Geometry check sheet. Reference: the model listing, model coordinates, mm. Face numbers are marked on the shaded views. A direction names the side the tool comes from. Give positions to 0.01 mm unless a question says otherwise; leave off trailing zeros. Loops run counter-clockwise (first coordinate to the right, second up) from the corner with the lowest first, then second, coordinate; pieces in that order, holes last. Notation, with made-up numbers: (15.5, 55.25) -> (58.5, 55.25) arc R16 ccw to (58.5, 69.25) -> close; hole circle Ø7 at (2.5, 76). An arc over 180 degrees is marked (long way). Answer as a JSON object with one key per item and string values.
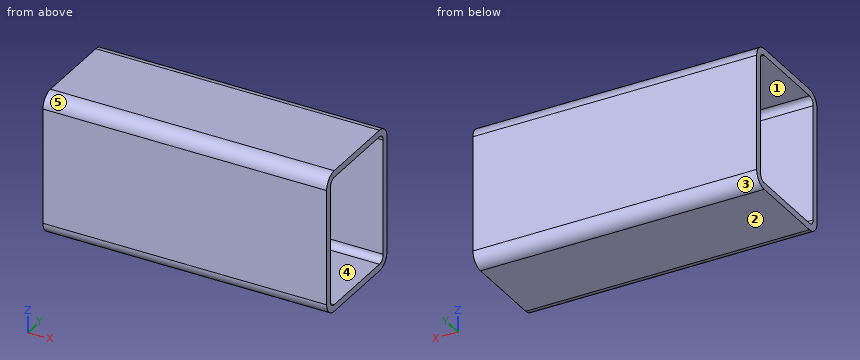
from build123d import *

# Parameters (mm, degrees)
F2_DEPTH = 101.6


# Not quite as in the source:
# - a variable given as a bare number and used for a length is read in inches; the dataset says mm whatever the document's units were


with BuildPart() as f2:
    # F1 (on Right) → F2 (new body, symmetric)
    with BuildSketch(Plane.YZ):
        with BuildLine():
            Line((28.575, 50.8), (-28.575, 50.8))
            ThreePointArc((-28.575, 50.8), (-35.3101920908, 48.0101920908), (-38.1, 41.275))
            Line((-38.1, 41.275), (-38.1, -41.275))
            ThreePointArc((-38.1, -41.275), (-35.3101920908, -48.0101920908), (-28.575, -50.8))
            Line((-28.575, -50.8), (28.575, -50.8))
            ThreePointArc((28.575, -50.8), (35.3101920908, -48.0101920908), (38.1, -41.275))
            Line((38.1, -41.275), (38.1, 41.275))
            ThreePointArc((38.1, 41.275), (35.3101920908, 48.0101920908), (28.575, 50.8))
        make_face()
        with BuildLine():
            ThreePointArc((-33.3375, 41.275), (-31.9425960454, 44.6425960454), (-28.575, 46.0375))
            Line((-28.575, 46.0375), (28.575, 46.0375))
            ThreePointArc((28.575, 46.0375), (31.9425960454, 44.6425960454), (33.3375, 41.275))
            Line((33.3375, 41.275), (33.3375, -41.275))
            ThreePointArc((33.3375, -41.275), (31.9425960454, -44.6425960454), (28.575, -46.0375))
            Line((28.575, -46.0375), (-28.575, -46.0375))
            ThreePointArc((-28.575, -46.0375), (-31.9425960454, -44.6425960454), (-33.3375, -41.275))
            Line((-33.3375, -41.275), (-33.3375, 41.275))
        make_face(mode=Mode.SUBTRACT)
    extrude(amount=F2_DEPTH, both=True)


solid = f2.part
1) Material ranges on line 1 along Y through (x, z) = (15.5, 22); line 2 along Z through (x, y) = (-57.5, -1.5); line 3 along Z through (x, y) = (6, -32), recorded low to high. Write a range as from..to.
Geometry check:
{"line 1": "y = -38.1..-33.34, 33.34..38.1", "line 2": "z = -50.8..-46.04, 46.04..50.8", "line 3": "z = -50.16..-44.58, 44.58..50.16"}
2) Depth check by flat-ended pin: P1, Ø4, axis at y = 29.5, z = -12, coming from the +X side. Enter the tip coordinate at first touch or a pass-through.
Geometry check:
{"P1": "passes through"}
3) Draft check along Y on the marked faces 1, 2 and 3. Enter one of: pulls with the +Y half, pulls with the -Y half, needs draft (parallel to the pull), parting line crosses it, or undercut.
Geometry check:
{"face 1": "undercut", "face 2": "needs draft", "face 3": "pulls with the +Y half"}
4) Section check B-B on y = -6. Record the cut outline in (x, z).
Geometry check:
{"outline": "(-101.6, -50.8) -> (101.6, -50.8) -> (101.6, -46.04) -> (-101.6, -46.04) -> close; (-101.6, 46.04) -> (101.6, 46.04) -> (101.6, 50.8) -> (-101.6, 50.8) -> close"}
5) Section check A-A on z = 16. Record the cut outline in (x, y), plus the area to 3 significant figures.
Geometry check:
{"outline": "(-101.6, -38.1) -> (101.6, -38.1) -> (101.6, -33.34) -> (-101.6, -33.34) -> close; (-101.6, 33.34) -> (101.6, 33.34) -> (101.6, 38.1) -> (-101.6, 38.1) -> close", "area": "1,940 mm2"}
6) Tool access check on the marked faces 4 and 5. Record the directions out of +Z, -Z, +X, -X, +Y, -Y that give a thin tool (end or side, any length) a straight path to the whole face; none if there is none.
Geometry check:
{"face 4": "+X, -X", "face 5": "+Z, +X, -X, -Y"}
